Here's how the part is built. I have some questions about the finished solid (model axes, mm). Face numbers are marked on the shaded views. A direction names the side the tool comes from. Give positions to 0.01 mm unless a question says otherwise; leave off trailing zeros. Order: outer loops, then holes, each group sorted by start corner. A loop starts at its lowest first (then second) coordinate and runs counter-clockwise, first axis right, second up.
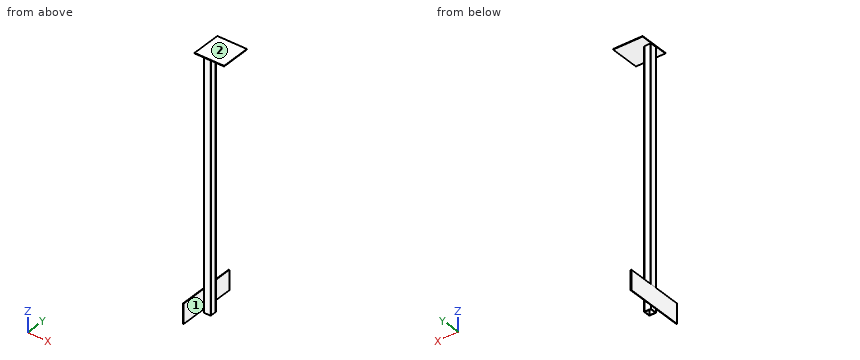
from build123d import *

# Parameters (mm, degrees)
F0_W     = 70
F0_H     = 2600
F1_DEPTH = 70
F2_W     = 60
F2_H     = 60
F3_DEPTH = 2600
F4_W     = 600
F4_H     = 200
F5_DEPTH = 6
F6_R     = 5
F7_W     = 300
F7_H     = 300
F8_DEPTH = 6


with BuildPart() as f1:
    # F0 (on Front) → F1 (new body)
    with BuildSketch(Plane.XZ):
        with Locations((-20.9116117656, 1237.1002838016)):
            Rectangle(F0_W, F0_H)
    extrude(amount=F1_DEPTH)

    # F2 (on face) → F3 (cut, through all)
    with BuildSketch(Plane(origin=(0, 0, -62.8997161984), x_dir=(1, 0, 0), z_dir=(0, 0, -1))):
        with Locations((-20.9116117656, 35)):
            Rectangle(F2_W, F2_H)
    extrude(amount=-F3_DEPTH, mode=Mode.SUBTRACT)

    # F4 (on face) → F5 (join)
    with BuildSketch(Plane(origin=(-55.9116117656, 0, 0), x_dir=(0, -1, 0), z_dir=(-1, 0, 0))):
        with Locations((35, 72.1002838016)):
            Rectangle(F4_W, F4_H)
    extrude(amount=F5_DEPTH)

    # F6
    f6_edges = [f1.edges().sort_by_distance(p)[0] for p in [
        (14.088388, 0, 1237.100284),
        (14.088388, -70, 1237.100284),
        (-55.911612, 0, 1354.600284),
        (-55.911612, -70, 1354.600284),
    ]]
    fillet(f6_edges, radius=F6_R)

    # F7 (on face) → F8 (join)
    with BuildSketch(Plane.XY.offset(2537.1002838016)):
        with Locations((89.0883882344, -35)):
            Rectangle(F7_W, F7_H)
    extrude(amount=F8_DEPTH)


solid = f1.part
Q1. If we section it at B-B on x = -17: List the corners of the cut face in (y, z) for me, plus the area to 3 significant figures.
Filled sheet:
outline: (-185, 2537.1) - (-70, 2537.1) - (-70, -62.9) - (-65, -62.9) - (-65, 2537.1) - (-5, 2537.1) - (-5, -62.9) - (0, -62.9) - (0, 2537.1) - (115, 2537.1) - (115, 2543.1) - (-185, 2543.1) - close
area: 27,800 mm2
Q2. If we section it at C-C on y = 168: List the corners of the cut face in (x, z) for me, plus the area to 3 significant figures.
Filled sheet:
outline: (-61.91, -27.9) - (-55.91, -27.9) - (-55.91, 172.1) - (-61.91, 172.1) - close
area: 1,200 mm2
Q3. I'm going to push flat-ended pins straight in: P1, Ø10, axis at x = 147.5, y = -1, coming from the -Z side; P2, Ø17.5, axis at y = -40.5, z = -38.5, coming from the -X side; P3, Ø18, axis at x = -16, z = 1077, coming from the +Y side. Where does each tip first touch, or does it pass through?
Filled sheet:
P1: stops at z = 2537.1
P2: stops at x = -55.91
P3: stops at y = 0
Q4. If we section it at A-A on z = 1574: List the corners of the cut face in (x, y) for me.
Filled sheet:
outline: (-55.91, -65) arc R5 ccw to (-50.91, -70) - (9.09, -70) arc R5 ccw to (14.09, -65) - (14.09, -5) arc R5 ccw to (9.09, 0) - (-50.91, 0) arc R5 ccw to (-55.91, -5) - close; hole (-50.91, -65) - (9.09, -65) - (9.09, -5) - (-50.91, -5) - close
Q5. I need wall thicknesses on L1, parallel to Y at x = -27.5, z = 1735.5; L2, parallel to X at y = -39, z = 1603; L3, parallel to Z at x = -11, y = -105.5. Which ranges of each line are inside material? Lowest first, please.
Filled sheet:
L1: y = -70 to -65, -5 to 0
L2: x = -55.91 to -50.91, 9.09 to 14.09
L3: z = 2537.1 to 2543.1
Q6. For the marked faces 1 and 2, which set-ups out of +Z, -Z, +X, -X, +Y, -Y let a thin tool reach every point of the face, with its end or its side?
Filled sheet:
face 1: -Z, +X, -Y
face 2: +Z, +X, -X, +Y, -Y
